```python
from build123d import *

# Parameters (mm, degrees)
BOSS_EXTRUDE1_START = -5.125
SKETCH1_W           = 32.8
SKETCH1_H           = 16.2
BOSS_EXTRUDE1_DEPTH = 10.275
CUT_EXTRUDE1_START  = -3.475
SKETCH2_W           = 23.2
SKETCH2_H           = 13
CUT_EXTRUDE1_DEPTH  = 8.625
CUT_EXTRUDE2_START  = 2.15
SKETCH3_R           = 1
CUT_EXTRUDE2_DEPTH  = 3
CUT_EXTRUDE3_START  = 2.15
SKETCH4_R           = 1
CUT_EXTRUDE3_DEPTH  = 3
CUT_EXTRUDE4_START  = -14.1
SKETCH5_R           = 3.15
CUT_EXTRUDE4_DEPTH  = 1.3
CUT_EXTRUDE5_START  = 14
SKETCH6_W           = 6
SKETCH6_H           = 4.4
CUT_EXTRUDE5_DEPTH  = 2.4


with BuildPart() as part:
    # Sketch1 → Boss-Extrude1 (new, symmetric)
    with BuildSketch(Plane.XY.offset(BOSS_EXTRUDE1_START)):
        Rectangle(SKETCH1_W, SKETCH1_H)
    extrude(amount=BOSS_EXTRUDE1_DEPTH, both=True)

    # Sketch2 → Cut-Extrude1 (cut, symmetric)
    with BuildSketch(Plane.XY.offset(CUT_EXTRUDE1_START)):
        Rectangle(SKETCH2_W, SKETCH2_H)
    extrude(amount=CUT_EXTRUDE1_DEPTH, both=True, mode=Mode.SUBTRACT)

    # Sketch3 → Cut-Extrude2 (cut, symmetric)
    with BuildSketch(Plane.XY.offset(CUT_EXTRUDE2_START)):
        with Locations((-13.75, 0)):
            Circle(SKETCH3_R)
    extrude(amount=CUT_EXTRUDE2_DEPTH, both=True, mode=Mode.SUBTRACT)

    # Sketch4 → Cut-Extrude3 (cut, symmetric)
    with BuildSketch(Plane.XY.offset(CUT_EXTRUDE3_START)):
        with Locations((13.75, 0)):
            Circle(SKETCH4_R)
    extrude(amount=CUT_EXTRUDE3_DEPTH, both=True, mode=Mode.SUBTRACT)

    # Sketch5 → Cut-Extrude4 (cut, symmetric)
    with BuildSketch(Plane.XY.offset(CUT_EXTRUDE4_START)):
        with Locations((5.5, 0)):
            Circle(SKETCH5_R)
    extrude(amount=CUT_EXTRUDE4_DEPTH, both=True, mode=Mode.SUBTRACT)

    # Sketch6 → Cut-Extrude5 (cut, symmetric)
    with BuildSketch(Plane(origin=(0, 0, 0), x_dir=(0, 0, -1), z_dir=(1, 0, 0)).offset(CUT_EXTRUDE5_START)):
        with Locations((9.1, 0)):
            Rectangle(SKETCH6_W, SKETCH6_H)
    extrude(amount=CUT_EXTRUDE5_DEPTH, both=True, mode=Mode.SUBTRACT)


solid = part.part
```
Model file for the job. Use its own axes, mm. A direction names the side the tool comes from. Give positions to 0.01 mm unless a question says otherwise; leave off trailing zeros. Write each loop counter-clockwise with the first axis right and the second up, starting at its lowest first coordinate (ties: lowest second). Pieces come first, ordered by that corner, then holes. Notation, with made-up numbers: (77.5, -33) - (101.5, -33) arc R17 cw to (101.5, 0) - close; hole circle Ø1 at (58, 43.5). An arc over 180 degrees is marked (long way). One line per question, with ' | ' between items. Start each with the question number.
(1) Pin check, flat tips, straight feed: P1, Ø1.2, axis at x = -13.75, y = 0, coming from the +Z side; P2, Ø5.5, axis at x = 5.5, y = 0, coming from the +Z side. Stop position of each tip, or through.
(2) 3-axis set-ups, long thin cutter, end or side, ignore diameter. For faces 4 (the face through (-16.4, 0, -5)), 5 (the face through (8.41, -1.21, -14.08)), 6 (the face through (14, 2.2, -9)), 7 (the face through (0, 0, -15.4)), 8 (the face through (14, 0, -0.85)): which of +Z, -Z, +X, -X, +Y, -Y reach the whole face in a straight line?
(3) Wall check: line 1 along Y through (x, z) = (-13.75, 1.45); line 2 along Z through (x, y) = (14, 0); line 3 along X through (y, z) = (4, -4.75). Give the ranges that are in metal, low to high. Write a range as from..to.
(4) Slice it at B-B on z = -5.5. Write the cut outline in (x, y).
(5) Two-plate mould, pull along Y, no slides. Class faces 1 (the face through (0, 8.1, -5)), 2 (the face through (14, 0, -6.1)), 3 (the face through (0, -7, 5.15)): +Y half, -Y half, draft (parallel to the pull), parting line (faces both ways), or undercut.
(6) Slice it at C-C on x = 13.75. Write the cut outline in (y, z), plus the area to 3 significant figures.
(7) Slice it at A-A on y = 0. Write the cut outline in (x, z), plus the area to 3 significant figures.
(8) Slice it at D-D on z = 1.5. Write the cut outline in (x, y), plus the area to 3 significant figures.
Results below:
1) P1: z = -0.85 | P2: z = -12.1
2) face 4: +Z, -Z, -X, +Y, -Y | face 5: -Z | face 6: +X | face 7: -Z, +X, -X, +Y, -Y | face 8: +Z
3) line 1: -8.1..-1, 1..8.1 | line 2: -15.4..-12.1, -6.1..-0.85 | line 3: -16.4..-11.6, 11.6..16.4
4) outline: (-16.4, -8.1) - (16.4, -8.1) - (16.4, 8.1) - (-16.4, 8.1) - close; hole (-11.6, -6.5) - (11.6, -6.5) - (11.6, 6.5) - (-11.6, 6.5) - close
5) face 1: +Y half | face 2: undercut | face 3: draft
6) outline: (-8.1, -15.4) - (8.1, -15.4) - (8.1, 5.15) - (1, 5.15) - (1, -0.85) - (-1, -0.85) - (-1, 5.15) - (-8.1, 5.15) - close; hole (-2.2, -12.1) - (2.2, -12.1) - (2.2, -6.1) - (-2.2, -6.1) - close | area: 295 mm^2
7) outline: (-16.4, -15.4) - (2.35, -15.4) - (2.35, -12.8) - (8.65, -12.8) - (8.65, -15.4) - (16.4, -15.4) - (16.4, -12.1) - (-11.6, -12.1) - (-11.6, 5.15) - (-12.75, 5.15) - (-12.75, -0.85) - (-14.75, -0.85) - (-14.75, 5.15) - (-16.4, 5.15) - close; (11.6, -6.1) - (16.4, -6.1) - (16.4, 5.15) - (14.75, 5.15) - (14.75, -0.85) - (12.75, -0.85) - (12.75, 5.15) - (11.6, 5.15) - close | area: 205 mm^2
8) outline: (-16.4, -8.1) - (16.4, -8.1) - (16.4, 8.1) - (-16.4, 8.1) - close; hole circle Ø2 at (-13.75, 0); hole (-11.6, -6.5) - (11.6, -6.5) - (11.6, 6.5) - (-11.6, 6.5) - close; hole circle Ø2 at (13.75, 0) | area: 223 mm^2
